```python
from build123d import *

# Parameters (mm, degrees)
SALIENTE_EXTRUIR1_DEPTH = 11
CROQUIS2_R              = 11
CORTAR_EXTRUIR1_DEPTH   = 7
CROQUIS3_R              = 19
SALIENTE_EXTRUIR2_DEPTH = 10
CROQUIS4_R              = 4
CORTAR_EXTRUIR2_DEPTH   = 18
SALIENTE_EXTRUIR3_DEPTH = 52
SALIENTE_EXTRUIR4_DEPTH = 11
CORTAR_EXTRUIR3_START   = -22
CROQUIS7_R              = 4
CORTAR_EXTRUIR3_DEPTH   = 22
SALIENTE_EXTRUIR5_START = 11
CROQUIS8_R              = 19
SALIENTE_EXTRUIR5_DEPTH = 11
CROQUIS10_R             = 4
CORTAR_EXTRUIR5_DEPTH   = 102.39773173
CORTAR_EXTRUIR6_START   = -7
CROQUIS11_R             = 11
CORTAR_EXTRUIR6_DEPTH   = 7
SALIENTE_EXTRUIR6_DEPTH = 10
SALIENTE_EXTRUIR7_START = 11
SALIENTE_EXTRUIR7_DEPTH = 11
CROQUIS14_R             = 2
CORTAR_EXTRUIR7_DEPTH   = 11
CORTAR_EXTRUIR8_DEPTH   = 4


with BuildPart() as part:
    # Croquis1 → Saliente-Extruir1 (new body)
    with BuildSketch(Plane.XY):
        with BuildLine():
            Line((-32.5, 0), (-25, -72.5))
            Line((-25, -72.5), (25, -72.5))
            Line((25, -72.5), (32.5, 0))
            ThreePointArc((32.5, 0), (0, 32.5), (-32.5, 0))
        make_face()
    extrude(amount=SALIENTE_EXTRUIR1_DEPTH)

    # Croquis2 → Cortar-Extruir1 (cut)
    with BuildSketch(Plane.XY.offset(11)):
        Circle(CROQUIS2_R)
    extrude(amount=-CORTAR_EXTRUIR1_DEPTH, mode=Mode.SUBTRACT)

    # Croquis3 → Saliente-Extruir2 (add)
    with BuildSketch(Plane(origin=(0, 0, 0), x_dir=(-1, 0, 0), z_dir=(0, 0, -1))):
        with Locations(Location((0, 0, 0), (0, 0, 180))):
            Circle(CROQUIS3_R)
    extrude(amount=SALIENTE_EXTRUIR2_DEPTH)

    # Croquis4 → Cortar-Extruir2 (cut)
    with BuildSketch(Plane.XY.offset(4)):
        Circle(CROQUIS4_R)
    extrude(amount=-CORTAR_EXTRUIR2_DEPTH, mode=Mode.SUBTRACT)

    # Croquis5 → Saliente-Extruir3 (add)
    with BuildSketch(Plane(origin=(0, 0, 0), x_dir=(-1, 0, 0), z_dir=(0, 0, -1))):
        Polygon((-25, -72.5), (25, -72.5), (26.034482759, -62.5), (-26.034482759, -62.5), align=None)
    extrude(amount=SALIENTE_EXTRUIR3_DEPTH)

    # Croquis6 → Saliente-Extruir4 (add)
    with BuildSketch(Plane(origin=(0, 0, -52), x_dir=(-1, 0, 0), z_dir=(0, 0, -1))):
        with BuildLine():
            Line((25, -72.5), (32.5, 0))
            ThreePointArc((32.5, 0), (0, 32.5), (-32.5, 0))
            Line((-32.5, 0), (-25, -72.5))
            Line((-25, -72.5), (25, -72.5))
        make_face()
    extrude(amount=-SALIENTE_EXTRUIR4_DEPTH)

    # Croquis7 → Cortar-Extruir3 (cut)
    with BuildSketch(Plane(origin=(0, 0, -52), x_dir=(-1, 0, 0), z_dir=(0, 0, -1)).offset(CORTAR_EXTRUIR3_START)):
        with Locations(Location((0, 0, 0), (0, 0, 180))):
            Circle(CROQUIS7_R)
    extrude(amount=CORTAR_EXTRUIR3_DEPTH, mode=Mode.SUBTRACT)

    # Croquis8 → Saliente-Extruir5 (add)
    with BuildSketch(Plane.XY.offset(-41).offset(SALIENTE_EXTRUIR5_START)):
        Circle(CROQUIS8_R)
    extrude(amount=-SALIENTE_EXTRUIR5_DEPTH)

    # Croquis10 → Cortar-Extruir5 (cut, through all)
    with BuildSketch(Plane(origin=(0, 0, -52), x_dir=(-1, 0, 0), z_dir=(0, 0, -1))):
        with Locations(Location((0, 0, 0), (0, 0, 180))):
            Circle(CROQUIS10_R)
    extrude(amount=-CORTAR_EXTRUIR5_DEPTH, mode=Mode.SUBTRACT)

    # Croquis11 → Cortar-Extruir6 (cut)
    with BuildSketch(Plane(origin=(0, 0, -52), x_dir=(-1, 0, 0), z_dir=(0, 0, -1)).offset(CORTAR_EXTRUIR6_START)):
        with Locations(Location((0, 0, 0), (0, 0, 180))):
            Circle(CROQUIS11_R)
    extrude(amount=CORTAR_EXTRUIR6_DEPTH, mode=Mode.SUBTRACT)

    # Croquis12 → Saliente-Extruir6 (add)
    with BuildSketch(Plane(origin=(0, 0, 0), x_dir=(-1, 0, 0), z_dir=(0, 0, -1))):
        with BuildLine():
            Line((-18.352590699, -4.917561857), (-28.011848962, -7.505752308))
            ThreePointArc((-28.011848962, -7.505752308), (-5.035797152, -28.559424837), (23.755409284, -16.633716654))
            Line((23.755409284, -16.633716654), (15.563888841, -10.897952291))
            ThreePointArc((15.563888841, -10.897952291), (-3.299315376, -18.711347307), (-18.352590699, -4.917561857))
        make_face()
    extrude(amount=SALIENTE_EXTRUIR6_DEPTH)

    # Croquis13 → Saliente-Extruir7 (add)
    with BuildSketch(Plane.XY.offset(-41).offset(SALIENTE_EXTRUIR7_START)):
        with BuildLine():
            Line((-15.563888841, -10.897952291), (-23.755409284, -16.633716654))
            ThreePointArc((-23.755409284, -16.633716654), (5.035797152, -28.559424837), (28.011848962, -7.505752308))
            Line((28.011848962, -7.505752308), (18.352590699, -4.917561857))
            ThreePointArc((18.352590699, -4.917561857), (3.299315376, -18.711347307), (-15.563888841, -10.897952291))
        make_face()
    extrude(amount=-SALIENTE_EXTRUIR7_DEPTH)

    # Croquis14 → Cortar-Extruir7 (cut)
    with BuildSketch(Plane(origin=(0, -62.5, 0), x_dir=(1, 0, 0), z_dir=(0, 1, 0))):
        with Locations(Location((-13, 30.5, 0), (0, 0, 270))):
            Circle(CROQUIS14_R)
        with Locations(Location((13, 30.5, 0), (0, 0, 270))):
            Circle(CROQUIS14_R)
        with Locations(Location((13, 10.5, 0), (0, 0, 270))):
            Circle(CROQUIS14_R)
        with Locations(Location((-13, 10.5, 0), (0, 0, 270))):
            Circle(CROQUIS14_R)
    extrude(amount=-CORTAR_EXTRUIR7_DEPTH, mode=Mode.SUBTRACT)

    # Croquis15 → Cortar-Extruir8 (cut)
    with BuildSketch(Plane(origin=(0, -62.5, 0), x_dir=(1, 0, 0), z_dir=(0, 1, 0))):
        Polygon((13, 26.458548116), (9.5, 28.479274058), (9.5, 32.520725942), (13, 34.541451884), (16.5, 32.520725942), (16.5, 28.479274058), align=None)
        Polygon((-9.5, 28.479274058), (-9.5, 32.520725942), (-13, 34.541451884), (-16.5, 32.520725942), (-16.5, 28.479274058), (-13, 26.458548116), align=None)
        Polygon((16.5, 12.520725942), (13, 14.541451884), (9.5, 12.520725942), (9.5, 8.479274058), (13, 6.458548116), (16.5, 8.479274058), align=None)
        Polygon((-13, 14.541451884), (-9.5, 12.520725942), (-9.5, 8.479274058), (-13, 6.458548116), (-16.5, 8.479274058), (-16.5, 12.520725942), align=None)
    extrude(amount=-CORTAR_EXTRUIR8_DEPTH, mode=Mode.SUBTRACT)


solid = part.part
```
Can you work these out from the model? Positions are in its coordinate system, mm. A direction names the side the tool comes from. Round coordinates to 2 decimals unless told otherwise and drop trailing zeros. Loops run counter-clockwise (first coordinate to the right, second up) from the corner with the lowest first, then second, coordinate; pieces in that order, holes last. Notation, with made-up numbers: M 69.25,44.25 L 80.25,44.25 A22 cw 80.25,78.25 Z; hole C 77,67.25 d3. An arc over 180 degrees is marked long. Answer as a JSON object with one key per item and string values. Group by question number.
Q1. Will these pins go through, and if not, where does the flat tip stop? pin 1 (1.2 mm diameter, centred on y = -64, z = -10, fed in from -X); pin 2 (20 mm diameter, centred on x = 0, y = 0, fed in from -Z); pin 3 (3 mm diameter, centred on x = 13, z = -10.5, fed in from +Y).
Q2. Imagine slicing it at A-A, the plane x = 0. Count the separate pieces of the cut face and the enclosed holes in it, then the cut area to 3 significant figures.
Q3. Please list where these lines run through material, in increasing order: L1, parallel to Z at x = 16, y = 9; L2, parallel to Z at x = 19.5, y = 15; L3, parallel to Y at x = 0, z = -2.75.
Q4. Imagine slicing it at D-D, the plane x = -28. Please give me the cut outline in (y, z).
Q5. Imagine slicing it at C-C, the plane y = -35. Please give me the cut outline in (x, z), then the cut area to 3 significant figures.
Q6. Imagine slicing it at B-B, the plane z = 6.5. Please give me the cut outline in (x, y), then the cut area to 3 significant figures.
Q7. We'd pull the mould along X, two halves only. Please class faces 1 (the flat face through (-11.2, -64.5, -7.5)), 2 (the flat face through (-11.2, -64.5, -33.5)), 3 (the flat face through (2, -5, -10)), 4 (the cylindrical face through (-0.715, 32.492, -46.577)): +X half, -X half, draft (parallel to the pull), parting line (faces both ways), or undercut.
Q8. On a 3-axis mill with a long thin cutter (end or side, diameter ignored), from which of +Z, -Z, +X, -X, +Y, -Y can I reach the whole of each face in a straight line? I mean faces 5 (the flat face through (0, -62.5, -20)), 6 (the cylindrical face through (-2.38, -10.74, 7.55)), 7 (the flat face through (9.5, -64, -30)), 8 (the flat face through (-14.8, -64.5, -27.5)). Say none if no direction works.
Findings:
{
 "1": {"pin 1": "stops at x = -25.94", "pin 2": "stops at z = -45", "pin 3": "stops at y = 15.06"},
 "2": {"separate pieces": "3", "enclosed holes": "0", "area": "3,190 mm2"},
 "3": {"L1": "z = -52 to -30, -10 to 11", "L2": "z = -52 to -41, 0 to 11", "L3": "y = -72.5 to -62.5, -29 to -4, 4 to 19"},
 "4": {"outline": "M -43.5,-52 L 16.5,-52 L 16.5,-41 L -43.5,-41 Z; M -43.5,0 L 16.5,0 L 16.5,11 L -43.5,11 Z"},
 "5": {"outline": "M -28.88,-52 L 28.88,-52 L 28.88,-41 L -28.88,-41 Z; M -28.88,0 L 28.88,0 L 28.88,11 L -28.88,11 Z", "area": "1,270 mm2"},
 "6": {"outline": "M -32.5,0 L -25,-72.5 L 25,-72.5 L 32.5,0 A32.5 ccw Z; hole C 0,0 d22", "area": "5,450 mm2"},
 "7": {"face 1": "undercut", "face 2": "undercut", "face 3": "draft", "face 4": "parting line"},
 "8": {"face 5": "+X, -X", "face 6": "+Z", "face 7": "none", "face 8": "+Y"}
}
